from build123d import *

# Parameters (mm, degrees)
EXTRUDE_THIN2_START                       = -25.4
EXTRUDE_THIN2_DEPTH                       = 25.4
BOSS_EXTRUDE1_START                       = -2.54
BOSS_EXTRUDE1_DEPTH                       = 2.54
BOSS_EXTRUDE2_DEPTH                       = 2.54
F_15_64_0_23438_DIAMETER_HOLE1_AT_2_COUNT = 2
F_15_64_0_23438_DIAMETER_HOLE1_AT_2_PITCH = 86.36
F_15_64_0_23438_DIAMETER_HOLE1_AT_3_COUNT = 2
F_15_64_0_23438_DIAMETER_HOLE1_AT_3_PITCH = 195.381977675
F_15_64_0_23438_DIAMETER_HOLE1_AT_4_COUNT = 2
F_15_64_0_23438_DIAMETER_HOLE1_AT_4_PITCH = 175.26


# Read off the part's stored shape, not the designer's step: Extrude-Thin2
with BuildPart() as part:
    # Extrude-Thin2 outline → Extrude-Thin2 (new body)
    with BuildSketch(Plane.XY.offset(EXTRUDE_THIN2_START)):
        with BuildLine():
            Line((-80.828024073, 36.556311377), (-80.828024073, 50.8))
            Line((-80.828024073, 50.8), (-87.63, 50.8))
            ThreePointArc((-87.63, 50.8), (-93.018153673, 48.568153673), (-95.25, 43.18))
            Line((-95.25, 43.18), (-95.25, -43.18))
            ThreePointArc((-95.25, -43.18), (-93.018153673, -48.568153673), (-87.63, -50.8))
            Line((-87.63, -50.8), (-80.828024073, -50.8))
            Line((-80.828024073, -50.8), (-80.828024073, -36.556311377))
            Line((-80.828024073, -36.556311377), (-52.888024073, -36.556311377))
            Line((-52.888024073, -36.556311377), (-52.888024073, -28.936311377))
            Line((-52.888024073, -28.936311377), (-40.188024073, -28.936311377))
            Line((-40.188024073, -28.936311377), (-40.188024073, -36.556311377))
            add(Edge.make_bspline(
                [(-40.188024073, -36.556311377), (6.000491779, -33.499243365), (9.490782471, -50.8)],
                knots=[0, 0, 0, 0.610951086, 0.610951086, 0.610951086], degree=2))
            Line((9.490782471, -50.8), (87.63, -50.8))
            ThreePointArc((87.63, -50.8), (93.018153673, -48.568153673), (95.25, -43.18))
            Line((95.25, -43.18), (95.25, 43.18))
            ThreePointArc((95.25, 43.18), (93.018153673, 48.568153673), (87.63, 50.8))
            Line((87.63, 50.8), (9.490782471, 50.8))
            add(Edge.make_bspline(
                [(9.490782471, 50.8), (6.000491779, 33.499243365), (-40.188024073, 36.556311377)],
                knots=[0, 0, 0, 0.610951086, 0.610951086, 0.610951086], degree=2))
            Line((-40.188024073, 36.556311377), (-40.188024073, 28.936311377))
            Line((-40.188024073, 28.936311377), (-52.888024073, 28.936311377))
            Line((-52.888024073, 28.936311377), (-52.888024073, 36.556311377))
            Line((-52.888024073, 36.556311377), (-80.828024073, 36.556311377))
        make_face()
        with BuildLine():
            Line((-87.63, 48.768), (-82.860024073, 48.768))
            Line((-82.860024073, 48.768), (-82.860024073, 34.524311377))
            Line((-82.860024073, 34.524311377), (-54.920024073, 34.524311377))
            Line((-54.920024073, 34.524311377), (-54.920024073, 26.904311377))
            Line((-54.920024073, 26.904311377), (-38.156024073, 26.904311377))
            Line((-38.156024073, 26.904311377), (-38.156024073, 34.395144422))
            add(Edge.make_bspline(
                [(11.059099877, 48.768), (10.705913599, 47.666821526), (10.231462505, 46.631478385), (9.34485534, 45.173434414), (9.020114118, 44.703275583), (8.31285443, 43.794325504), (7.932752955, 43.359154617), (6.738556789, 42.126829372), (5.863761314, 41.393125544), (4.455909096, 40.399393999), (3.970643089, 40.086351658), (2.987111557, 39.50137004), (2.48684241, 39.227961499), (0.964119528, 38.456915884), (-0.080085669, 38.008090834), (-1.679731191, 37.409665787), (-2.218549861, 37.222765467), (-3.306137501, 36.871294096), (-3.856031524, 36.7064305), (-6.610131831, 35.936843126), (-8.830751105, 35.489873067), (-13.293085078, 34.801180583), (-15.535017784, 34.561579267), (-20.033665755, 34.226203327), (-22.290452983, 34.13112888), (-26.815059954, 34.048320676), (-29.084850225, 34.060938072), (-33.62255889, 34.169687173), (-35.889894754, 34.26582406), (-38.156024073, 34.395144422)],
                knots=[0, 0, 0, 0, 0.0625, 0.0625, 0.09375, 0.09375, 0.125, 0.125, 0.1875, 0.1875, 0.21875, 0.21875, 0.25, 0.25, 0.3125, 0.3125, 0.34375, 0.34375, 0.375, 0.375, 0.5, 0.5, 0.625, 0.625, 0.75, 0.75, 0.875, 0.875, 1, 1, 1, 1], degree=3))
            Line((11.059099877, 48.768), (87.63, 48.768))
            ThreePointArc((87.63, 48.768), (91.581312693, 47.131312693), (93.218, 43.18))
            Line((93.218, 43.18), (93.218, -43.18))
            ThreePointArc((93.218, -43.18), (91.581312693, -47.131312693), (87.63, -48.768))
            Line((87.63, -48.768), (11.059099877, -48.768))
            add(Edge.make_bspline(
                [(-38.156024073, -34.395144422), (-35.889212951, -34.265785152), (-33.622237618, -34.169696181), (-29.087874945, -34.060993864), (-26.820488385, -34.048222574), (-23.419006743, -34.110473753), (-22.285112177, -34.144870035), (-20.017166217, -34.245437307), (-18.881979516, -34.311696432), (-15.488251882, -34.56581331), (-13.239736034, -34.807790371), (-8.782595463, -35.498966347), (-6.573640775, -35.946451198), (-3.306890482, -36.860175418), (-2.225854522, -37.205688462), (-0.62007844, -37.805919033), (-0.086320204, -38.02031336), (0.963955056, -38.476496538), (1.481482977, -38.71859586), (3.008182433, -39.492540914), (3.991806837, -40.071413071), (5.399027077, -41.06529203), (5.854721193, -41.41662922), (6.723566444, -42.153236805), (7.138582961, -42.539781101), (8.320387349, -43.758860403), (9.024746312, -44.65099332), (10.229082778, -46.623668325), (10.706098691, -47.667398611), (11.059099877, -48.768)],
                knots=[0, 0, 0, 0, 0.125, 0.125, 0.25, 0.25, 0.3125, 0.3125, 0.375, 0.375, 0.5, 0.5, 0.625, 0.625, 0.6875, 0.6875, 0.71875, 0.71875, 0.75, 0.75, 0.8125, 0.8125, 0.84375, 0.84375, 0.875, 0.875, 0.9375, 0.9375, 1, 1, 1, 1], degree=3))
            Line((-38.156024073, -34.395144422), (-38.156024073, -26.904311377))
            Line((-38.156024073, -26.904311377), (-54.920024073, -26.904311377))
            Line((-54.920024073, -26.904311377), (-54.920024073, -34.524311377))
            Line((-54.920024073, -34.524311377), (-82.860024073, -34.524311377))
            Line((-82.860024073, -34.524311377), (-82.860024073, -48.768))
            Line((-82.860024073, -48.768), (-87.63, -48.768))
            ThreePointArc((-87.63, -48.768), (-91.581312693, -47.131312693), (-93.218, -43.18))
            Line((-93.218, -43.18), (-93.218, 43.18))
            ThreePointArc((-93.218, 43.18), (-91.581312693, 47.131312693), (-87.63, 48.768))
        make_face(mode=Mode.SUBTRACT)
    extrude(amount=EXTRUDE_THIN2_DEPTH)

    # Sketch11<2> → Boss-Extrude1 (add)
    with BuildSketch(Plane.XY.offset(BOSS_EXTRUDE1_START)):
        with BuildLine():
            Line((-80.828024073, 50.8), (-80.828024073, 36.556311377))
            Line((-80.828024073, 36.556311377), (-52.888024073, 36.556311377))
            Line((-52.888024073, 36.556311377), (-52.888024073, 28.936311377))
            Line((-52.888024073, 28.936311377), (-40.188024073, 28.936311377))
            Line((-40.188024073, 28.936311377), (-40.188024073, 36.556311377))
            add(Edge.make_bspline(
                [(-40.188024073, 36.556311377), (6.000491779, 33.499243365), (9.490782471, 50.8)],
                knots=[0, 0, 0, 0.610951086, 0.610951086, 0.610951086], degree=2))
            Line((9.490782471, 50.8), (87.63, 50.8))
            ThreePointArc((87.63, 50.8), (93.018153673, 48.568153673), (95.25, 43.18))
            Line((95.25, 43.18), (95.25, -43.18))
            ThreePointArc((95.25, -43.18), (93.018153673, -48.568153673), (87.63, -50.8))
            Line((87.63, -50.8), (9.490782471, -50.8))
            add(Edge.make_bspline(
                [(-40.188024073, -36.556311377), (6.000491779, -33.499243365), (9.490782471, -50.8)],
                knots=[0, 0, 0, 0.610951086, 0.610951086, 0.610951086], degree=2))
            Line((-40.188024073, -36.556311377), (-40.188024073, -28.936311377))
            Line((-40.188024073, -28.936311377), (-52.888024073, -28.936311377))
            Line((-52.888024073, -28.936311377), (-52.888024073, -36.556311377))
            Line((-52.888024073, -36.556311377), (-80.828024073, -36.556311377))
            Line((-80.828024073, -36.556311377), (-80.828024073, -50.8))
            Line((-80.828024073, -50.8), (-87.63, -50.8))
            ThreePointArc((-87.63, -50.8), (-93.018153673, -48.568153673), (-95.25, -43.18))
            Line((-95.25, -43.18), (-95.25, 43.18))
            ThreePointArc((-95.25, 43.18), (-93.018153673, 48.568153673), (-87.63, 50.8))
            Line((-87.63, 50.8), (-80.828024073, 50.8))
        make_face()
    extrude(amount=BOSS_EXTRUDE1_DEPTH)

    # Sketch14 → Boss-Extrude2 (add)
    with BuildSketch(Plane(origin=(0, 0, -25.4), x_dir=(-1, 0, 0), z_dir=(0, 0, -1))):
        with BuildLine():
            ThreePointArc((-95.25, -43.18), (-93.018153673, -48.568153673), (-87.63, -50.8))
            Line((-87.63, -50.8), (-81.532541243, -50.8))
            Line((-81.532541243, -50.8), (-81.532541243, -36.556311377))
            Line((-81.532541243, -36.556311377), (-95.25, -36.556311377))
            Line((-95.25, -36.556311377), (-95.25, -43.18))
        make_face()
        with BuildLine():
            Line((-95.25, 43.18), (-95.25, 36.556311377))
            Line((-95.25, 36.556311377), (-81.532541243, 36.556311377))
            Line((-81.532541243, 36.556311377), (-81.532541243, 50.8))
            Line((-81.532541243, 50.8), (-87.63, 50.8))
            ThreePointArc((-87.63, 50.8), (-93.018153673, 48.568153673), (-95.25, 43.18))
        make_face()
        with BuildLine():
            Line((95.25, -43.18), (95.25, -36.556311377))
            Line((95.25, -36.556311377), (80.828024073, -36.556311377))
            Line((80.828024073, -36.556311377), (80.828024073, -50.8))
            Line((80.828024073, -50.8), (87.63, -50.8))
            ThreePointArc((87.63, -50.8), (93.018153673, -48.568153673), (95.25, -43.18))
        make_face()
        with BuildLine():
            Line((87.63, 50.8), (80.828024073, 50.8))
            Line((80.828024073, 50.8), (80.828024073, 36.556311377))
            Line((80.828024073, 36.556311377), (95.25, 36.556311377))
            Line((95.25, 36.556311377), (95.25, 43.18))
            ThreePointArc((95.25, 43.18), (93.018153673, 48.568153673), (87.63, 50.8))
        make_face()
    extrude(amount=-BOSS_EXTRUDE2_DEPTH)

    # Sketch15 → 15/64 (0.23438) Diameter Hole1 (revolve, cut)
    with BuildSketch(Plane(origin=(87.63, 43.18, -25.4), x_dir=(0, 1, 0), z_dir=(1, 0, 0))):
        Polygon((0, 0), (0, 2.54), (2.976626, 2.54), (2.976626, 0.532828266), (3.611626, 0), align=None)
    f_15_64_0_23438_diameter_hole1 = revolve(axis=Axis((87.63, 43.18, -31.75), (0, 0, 1)), mode=Mode.SUBTRACT)

    # 15/64 (0.23438) Diameter Hole1 at 2: 15/64 (0.23438) Diameter Hole1 ×2
    with Locations(*[(0, -i * F_15_64_0_23438_DIAMETER_HOLE1_AT_2_PITCH, 0) for i in range(1, F_15_64_0_23438_DIAMETER_HOLE1_AT_2_COUNT)]):
        add(f_15_64_0_23438_diameter_hole1, mode=Mode.SUBTRACT)

    # 15/64 (0.23438) Diameter Hole1 at 3: 15/64 (0.23438) Diameter Hole1 ×2
    with Locations(*[Vector(-0.8970121097452229, -0.44200596712083456, 0) * (i * F_15_64_0_23438_DIAMETER_HOLE1_AT_3_PITCH) for i in range(1, F_15_64_0_23438_DIAMETER_HOLE1_AT_3_COUNT)]):
        add(f_15_64_0_23438_diameter_hole1, mode=Mode.SUBTRACT)

    # 15/64 (0.23438) Diameter Hole1 at 4: 15/64 (0.23438) Diameter Hole1 ×2
    with Locations(*[(-i * F_15_64_0_23438_DIAMETER_HOLE1_AT_4_PITCH, 0, 0) for i in range(1, F_15_64_0_23438_DIAMETER_HOLE1_AT_4_COUNT)]):
        add(f_15_64_0_23438_diameter_hole1, mode=Mode.SUBTRACT)


solid = part.part
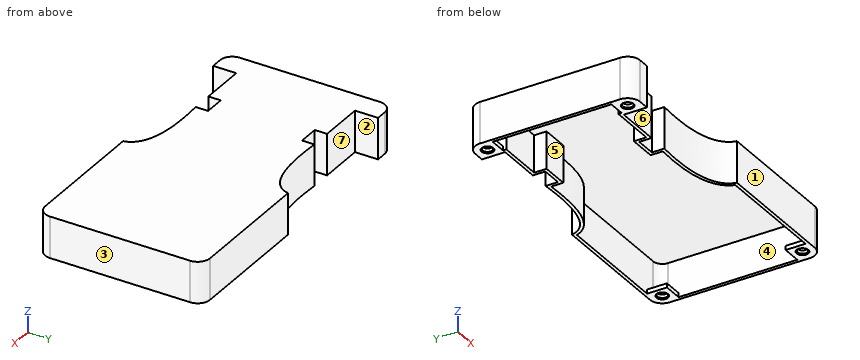
Source: CAD feature listing. Evaluate the final solid. Frame: model axes, mm. Face numbers are marked on the shaded views. A direction names the side the tool comes from. Give positions to 0.01 mm unless a question says otherwise; leave off trailing zeros. Write each loop counter-clockwise with the first axis right and the second up, starting at its lowest first coordinate (ties: lowest second). Pieces come first, ordered by that corner, then holes. Notation, with made-up numbers: M 89.25,32 L 128.25,32 A18 ccw 128.25,36 Z; hole C 53.25,-30.5 d9. An arc over 180 degrees is marked long. Return JSON: item names as keys, results as strings. Group by question number.
1) Cut plane A-A, the plane x = 46.5. Output: boundary loops of the cut face in (y, z), then the cut area to 3 significant figures.
2) Cut plane B-B, the plane y = 14.5. Output: boundary loops of the cut face in (x, z), then the cut area to 3 significant figures.
3) First-contact query: pin 1 Ø1 at (x, z) = (-42, -10) entering from -Y; pin 2 Ø8.5 at (x, z) = (-48, -9.5) entering from +Y; pin 3 Ø4 at (x, z) = (-6, -14.5) entering from +Y; pin 4 Ø11.5 at (y, z) = (-47, -9) entering from +X. Flat tips, straight axial feed; report the tip coordinate or a pass-through.
4) Set-up query: the marked faces 4, 5, 6 and 7. Return all of +Z, -Z, +X, -X, +Y, -Y with unobstructed straight access to the full face (end or side cutting, diameter ignored); none if empty.
5) Ray query, L1, parallel to X at y = 33, z = -15.25; L2, parallel to Y at x = 87.63, z = -23.75; L3, parallel to X at y = 27, z = -17.75. Return the intervals inside material, ascending.
6) Draft query along X for the marked faces 1, 2 and 3. Return one class per face: released by +X, released by -X, zero draft, split by the parting line, or undercut.
Data:
{
 "1": {"outline": "M -50.8,-25.4 L -48.77,-25.4 L -48.77,-2.54 L 48.77,-2.54 L 48.77,-25.4 L 50.8,-25.4 L 50.8,0 L -50.8,0 Z", "area": "351 mm²"},
 "2": {"outline": "M -95.25,-25.4 L -93.22,-25.4 L -93.22,-2.54 L 93.22,-2.54 L 93.22,-25.4 L 95.25,-25.4 L 95.25,0 L -95.25,0 Z", "area": "577 mm²"},
 "3": {"pin 1": "stops at y = -28.94", "pin 2": "stops at y = 28.94", "pin 3": "stops at y = 38.79", "pin 4": "stops at x = 95.25"},
 "4": {"face 4": "none", "face 5": "-Z", "face 6": "+Z, -Z, -Y", "face 7": "+Z, -Z, +Y"},
 "5": {"L1": "x = -95.25 to -93.22, -54.92 to -52.89, -40.19 to -38.16, 93.22 to 95.25", "L2": "y = -50.8 to -46.16, -40.2 to -36.56, 36.56 to 40.2, 46.16 to 50.8", "L3": "x = -95.25 to -93.22, -54.92 to -38.16, 93.22 to 95.25"},
 "6": {"face 1": "zero draft", "face 2": "undercut", "face 3": "released by +X"}
}
